CAD build for the part. Positions are in the model's coordinates, mm. Face numbers are marked on the shaded views. A direction names the side the tool comes from. Coordinates: 2 decimals unless noted, no trailing zeros. Loops run counter-clockwise (first coordinate to the right, second up) from the corner with the lowest first, then second, coordinate; pieces in that order, holes last. Notation, with made-up numbers: (85.5, 81.5) -> (144.5, 81.5) arc R23 cw to (144.5, 95.5) -> close; hole circle Ø8 at (45, -29). An arc over 180 degrees is marked (long way). Return JSON: item names as keys, results as strings. Group by question number.
(1) Mould opens along Z. For the marked faces 1, 2 and 3 say: pulls with the +Z half, pulls with the -Z half, needs draft (parallel to the pull), parting line crosses it, or undercut.
(2) Tool access for the marked faces 4 and 5: list every direction of +Z, -Z, +X, -X, +Y, -Y with a clear straight run to the whole face (end or side of a thin tool).
(3) Saw through at D-D on z = -4.5. Write the cut outline in (x, y).
(4) Probe L1, parallel to Z at x = -4, y = 6.5; L2, parallel to Y at x = -4.5, z = -4.5; L3, parallel to X at y = 8, z = -7. List the from-to ranges inside material, lowest first.
(5) Saw through at B-B on z = -1.5. Write the cut outline in (x, y), then the cut area to 3 significant figures.
(6) Saw through at A-A on x = -3.5. Write the cut outline in (y, z).
(7) Saw through at C-C on y = 6.5. Write the cut outline in (x, z).
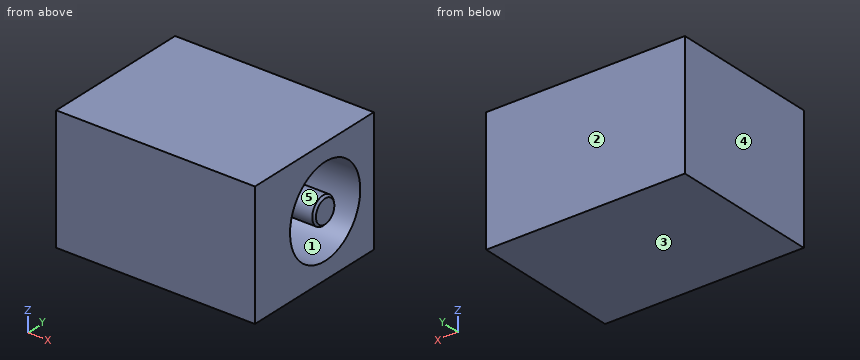
Autodesk Inventor part; units mm, degrees
ref_plane "YZ Plane" through (0, 0, 0) normal (1, 0, 0) x (0, 1, 0)
ref_plane "XZ Plane" through (0, 0, 0) normal (0, 1, 0) x (-1, 0, 0)
ref_plane "XY Plane" through (0, 0, 0) normal (0, 0, 1) x (1, 0, 0)
sketch "Szkic1" plane through (0, 0, 0) normal (0, 1, 0) x (-1, 0, 0)
  line L0 (14.4, -9) -> (0, -9)
  line L1 (0, -9) -> (0, 0)
  line L2 (0, 0) -> (14.4, 0)
  line L3 (14.4, 0) -> (14.4, -9)
  dimension "d0" = 9
  dimension "d1" = 14.4
extrude "Wyciągnięcie proste1" add sketch "Szkic1" along normal blind 11
sketch "Szkic2" plane through (0, 0, 0) normal (1, 0, 0) x (0, 0, -1)
  line L0 (0, 11) -> (9, 11)
  line L1 (4.5, 11) -> (4.5, 0)
  line L2 (0, 0) -> (9, 0)
  circle A0 centre (4.5, 6.5) radius 1
  circle A1 centre (4.5, 6.5) radius 3.25
  dimension "d4" = 2
  dimension "d5" = 6.5
  dimension "d6" = 6.5
extrude "Wyciągnięcie proste2" cut sketch "Szkic2" against normal blind 7 contours A1 L1 A0 | L1 A0 A1
chamfer "Faza1" distance 0.15 angle 45 1 edges at (0, 6.5, -3.5)
equation "\"d0\" = input_a"
equation "\"d1\" = input_b"
equation "\"d2\" = input_wys"
equation "\"gniazdo_M2_glebokosc\" = 1.5"
equation "\"gniazdo_M2_D1\" = 4.5"
equation "\"gniazdo_M2_D2\" = 2.6"
equation "\"insert_D\" = 2.4"
equation "\"insert_glebokosc\" = 5.5"
equation "\"podstawa_b\" = 65"
equation "\"podstawa_wys\" = 2"
equation "\"podstawa_otwory_montazowe_poz_x\" = 4"
equation "\"podstawa_otwory_montazowe_poz_y\" = 4"
equation "\"podstawa_zaokraglenie\" = 3"
equation "\"obudowa_b\" = 65"
equation "\"obudowa_wys\" = 36"
equation "\"obudowa_grubosc\" = 2"
equation "\"obudowa_kontrolki_a\" = 38"
equation "\"obudowa_otwory_montazowe_poz_x\" = 4"
equation "\"obudowa_otwory_montazowe_poz_y\" = 4"
equation "\"obudowa_otwory_montazowe_material_x\" = 8"
equation "\"obudowa_otwory_montazowe_material_y\" = 8"
equation "\"obudowa_zaokraglenie\" = 3"
equation "\"obudowa_otwory_io1_D\" = 11.5"
equation "\"obudowa_otwory_io1_wys\" = 15"
equation "\"obudowa_otwory_io2_D\" = 11.5"
equation "\"obudowa_otwory_io2_wys\" = 15"
equation "\"obudowa_otwory_pot_D\" = 8"
equation "\"input_a\" = 9"
equation "\"input_b\" = 14.4"
equation "\"input_wys\" = 11"
properties part number "9V_input" material "Polipropylen"
Geometry results:
{
 "1": {"face 1": "undercut", "face 2": "needs draft", "face 3": "pulls with the -Z half"},
 "2": {"face 4": "+Z, -Z, -X, +Y, -Y", "face 5": "+X"},
 "3": {"outline": "(-14.4, 0) -> (0, 0) -> (0, 3.25) -> (-7, 3.25) -> (-7, 5.5) -> (-0.15, 5.5) -> (0, 5.65) -> (0, 7.35) -> (-0.15, 7.5) -> (-7, 7.5) -> (-7, 9.75) -> (0, 9.75) -> (0, 11) -> (-14.4, 11) -> close"},
 "4": {"L1": "-9 to -7.75, -5.5 to -3.5, -1.25 to 0", "L2": "0 to 3.25, 5.5 to 7.5, 9.75 to 11", "L3": "-14.4 to -7"},
 "5": {"outline": "(-14.4, 0) -> (0, 0) -> (0, 5.25) -> (-7, 5.25) -> (-7, 7.75) -> (0, 7.75) -> (0, 11) -> (-14.4, 11) -> close", "area": "141 mm²"},
 "6": {"outline": "(0, -9) -> (11, -9) -> (11, 0) -> (0, 0) -> close; circle Ø2 at (6.5, -4.5); hole circle Ø6.5 at (6.5, -4.5)"},
 "7": {"outline": "(-14.4, -9) -> (0, -9) -> (0, -7.75) -> (-7, -7.75) -> (-7, -5.5) -> (-0.15, -5.5) -> (0, -5.35) -> (0, -3.65) -> (-0.15, -3.5) -> (-7, -3.5) -> (-7, -1.25) -> (0, -1.25) -> (0, 0) -> (-14.4, 0) -> close"}
}
